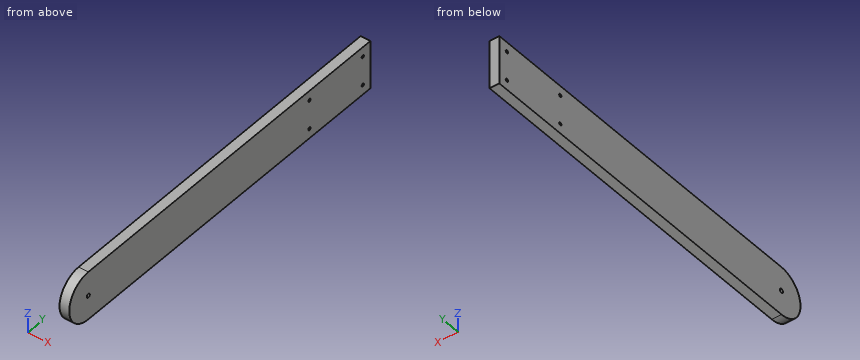
from build123d import *

# Parameters (mm, degrees)
BOSS_EXTRUDE2_DEPTH = 5
SKETCH4_R           = 0.75
CUT_EXTRUDE1_DEPTH  = 5
SKETCH5_R           = 1
CUT_EXTRUDE2_DEPTH  = 5


with BuildPart() as part:
    # Sketch3 → Boss-Extrude2 (new body)
    with BuildSketch(Plane(origin=(0, 0, 0), x_dir=(0, 0, -1), z_dir=(1, 0, 0))):
        with BuildLine():
            Line((12.5, 100), (-12.5, 100))
            Line((-12.5, 100), (-12.5, -85))
            ThreePointArc((-12.5, -85), (0, -97.5), (12.5, -85))
            Line((12.5, -85), (12.5, 100))
        make_face()
    extrude(amount=BOSS_EXTRUDE2_DEPTH)

    # Sketch4 → Cut-Extrude1 (cut)
    with BuildSketch(Plane.ZY):
        with Locations((-7.5, 95)):
            Circle(SKETCH4_R)
        with Locations(Location((-7.5, 60, 0), (0, 0, 180))):
            Circle(SKETCH4_R)
        with Locations((7.5, 60)):
            Circle(SKETCH4_R)
        with Locations(Location((7.5, 95, 0), (0, 0, 180))):
            Circle(SKETCH4_R)
    extrude(amount=-CUT_EXTRUDE1_DEPTH, mode=Mode.SUBTRACT)

    # Sketch5 → Cut-Extrude2 (cut)
    with BuildSketch(Plane.ZY):
        with Locations((0, -85)):
            Circle(SKETCH5_R)
    extrude(amount=-CUT_EXTRUDE2_DEPTH, mode=Mode.SUBTRACT)


solid = part.part
Check sheet for the modelled part. Datum: model origin and axes. Units: mm. Coordinates: 2 decimals unless noted, no trailing zeros. Write each loop counter-clockwise with the first axis right and the second up, starting at its lowest first coordinate (ties: lowest second). Pieces come first, ordered by that corner, then holes.
Item 1: Cross-section at A-A on x = 1.65. Record the boundary of the cut face in (y, z), then the cut area to 3 significant figures.
Numbers:
outline: (-85, -12.5) - (100, -12.5) - (100, 12.5) - (-85, 12.5) arc R12.5 ccw to start; hole circle Ø2 at (-85, 0); hole circle Ø1.5 at (60, -7.5); hole circle Ø1.5 at (60, 7.5); hole circle Ø1.5 at (95, -7.5); hole circle Ø1.5 at (95, 7.5)
area: 4,860 mm2
Item 2: Scan lines: probe 1 along Z at (x, y) = (2.7, 95); probe 2 along Y at (x, z) = (1.3, 7.5); probe 3 along Y at (x, z) = (1.9, -8). Record each from-to range of solid material in increasing order.
Numbers:
probe 1: z = -12.5 to -8.25, -6.75 to 6.75, 8.25 to 12.5
probe 2: y = -95 to 59.25, 60.75 to 94.25, 95.75 to 100
probe 3: y = -94.6 to 59.44, 60.56 to 94.44, 95.56 to 100
Item 3: Depth check by flat-ended pin: pin 1 Ø1.2 at (y, z) = (-85, 0) entering from +X. Enter the tip coordinate at first touch or a pass-through.
Numbers:
pin 1: passes through
